from build123d import *

# Parameters (mm, degrees)
F0_R       = 8.5
F1_DEPTH   = 3
F2_SIZE2   = 3
F2_SIZE    = 1.45
F2_2_SIZE2 = 3
F2_2_SIZE  = 1.45
F2_3_SIZE2 = 3
F2_3_SIZE  = 1.45
F2_4_SIZE2 = 3
F2_4_SIZE  = 1.45
F2_5_SIZE2 = 3
F2_5_SIZE  = 1.45
F2_6_SIZE2 = 3
F2_6_SIZE  = 1.45
F2_7_SIZE2 = 3
F2_7_SIZE  = 1.45
F2_8_SIZE2 = 3
F2_8_SIZE  = 1.45
F3_SIZE2   = 1.45
F3_SIZE    = 3


with BuildPart() as f1:
    # F0 (on Top) → F1 (new body)
    with BuildSketch(Plane.XY):
        Polygon((9.5147186258, 10.9705627485), (-1.0294372515, 14.4852813742), (-10.9705627485, 9.5147186258), (-14.4852813742, -1.0294372515), (-9.5147186258, -10.9705627485), (1.0294372515, -14.4852813742), (10.9705627485, -9.5147186258), (14.4852813742, 1.0294372515), align=None)
        Circle(F0_R, mode=Mode.SUBTRACT)
        Polygon((-9.5147186258, -10.9705627485), (-14.4852813742, -1.0294372515), (-21.2132034356, -21.2132034356), (-10.6066017178, -10.6066017178), align=None)
        Polygon((1.0294372515, -14.4852813742), (-9.5147186258, -10.9705627485), (0, -30), (0, -15), align=None)
        Polygon((10.6066017178, -10.6066017178), (10.9705627485, -9.5147186258), (1.0294372515, -14.4852813742), (21.2132034356, -21.2132034356), align=None)
        Polygon((15, 0), (14.4852813742, 1.0294372515), (10.9705627485, -9.5147186258), (30, 0), align=None)
        Polygon((10.6066017178, 10.6066017178), (9.5147186258, 10.9705627485), (14.4852813742, 1.0294372515), (21.2132034356, 21.2132034356), align=None)
        Polygon((0, 30), (0, 15), (-1.0294372515, 14.4852813742), (9.5147186258, 10.9705627485), align=None)
        Polygon((-10.9705627485, 9.5147186258), (-1.0294372515, 14.4852813742), (-21.2132034356, 21.2132034356), (-10.6066017178, 10.6066017178), align=None)
        Polygon((-14.4852813742, -1.0294372515), (-10.9705627485, 9.5147186258), (-30, 0), (-15, 0), align=None)
    extrude(amount=F1_DEPTH)

    # F2
    f2_edges = [f1.edges().sort_by_distance(p)[0] for p in [
        (-15.909903, 15.909903, 3),
    ]]
    f2_side = f1.faces().sort_by_distance((-15.909903, 15.909903, 1.5))[0]
    chamfer(f2_edges, length=F2_SIZE, length2=F2_SIZE2, reference=f2_side)

    # F2#2
    f2_2_edges = [f1.edges().sort_by_distance(p)[0] for p in [
        (-22.5, 0, 3),
    ]]
    f2_2_side = f1.faces().sort_by_distance((-22.5, 0, 1.5))[0]
    chamfer(f2_2_edges, length=F2_2_SIZE, length2=F2_2_SIZE2, reference=f2_2_side)

    # F2#3
    f2_3_edges = [f1.edges().sort_by_distance(p)[0] for p in [
        (-15.909903, -15.909903, 3),
    ]]
    f2_3_side = f1.faces().sort_by_distance((-15.909903, -15.909903, 1.5))[0]
    chamfer(f2_3_edges, length=F2_3_SIZE, length2=F2_3_SIZE2, reference=f2_3_side)

    # F2#4
    f2_4_edges = [f1.edges().sort_by_distance(p)[0] for p in [
        (0, -22.5, 3),
    ]]
    f2_4_side = f1.faces().sort_by_distance((0, -22.5, 1.5))[0]
    chamfer(f2_4_edges, length=F2_4_SIZE, length2=F2_4_SIZE2, reference=f2_4_side)

    # F2#5
    f2_5_edges = [f1.edges().sort_by_distance(p)[0] for p in [
        (15.909903, -15.909903, 3),
    ]]
    f2_5_side = f1.faces().sort_by_distance((15.909903, -15.909903, 1.5))[0]
    chamfer(f2_5_edges, length=F2_5_SIZE, length2=F2_5_SIZE2, reference=f2_5_side)

    # F2#6
    f2_6_edges = [f1.edges().sort_by_distance(p)[0] for p in [
        (22.5, 0, 3),
    ]]
    f2_6_side = f1.faces().sort_by_distance((22.5, 0, 1.5))[0]
    chamfer(f2_6_edges, length=F2_6_SIZE, length2=F2_6_SIZE2, reference=f2_6_side)

    # F2#7
    f2_7_edges = [f1.edges().sort_by_distance(p)[0] for p in [
        (15.909903, 15.909903, 3),
    ]]
    f2_7_side = f1.faces().sort_by_distance((15.909903, 15.909903, 1.5))[0]
    chamfer(f2_7_edges, length=F2_7_SIZE, length2=F2_7_SIZE2, reference=f2_7_side)

    # F2#8
    f2_8_edges = [f1.edges().sort_by_distance(p)[0] for p in [
        (0, 22.5, 3),
    ]]
    f2_8_side = f1.faces().sort_by_distance((0, 22.5, 1.5))[0]
    chamfer(f2_8_edges, length=F2_8_SIZE, length2=F2_8_SIZE2, reference=f2_8_side)

    # F3
    f3_edges = [f1.edges().sort_by_distance(p)[0] for p in [
        (0, -22.5, 0),
        (15.909903, -15.909903, 0),
        (22.5, 0, 0),
        (15.909903, 15.909903, 0),
        (0, 22.5, 0),
        (-15.909903, 15.909903, 0),
        (-22.5, 0, 0),
        (-15.909903, -15.909903, 0),
    ]]
    f3_side = f1.faces().sort_by_distance((-16.509903, -15.309903, 0))[0]
    chamfer(f3_edges, length=F3_SIZE, length2=F3_SIZE2, reference=f3_side)


solid = f1.part
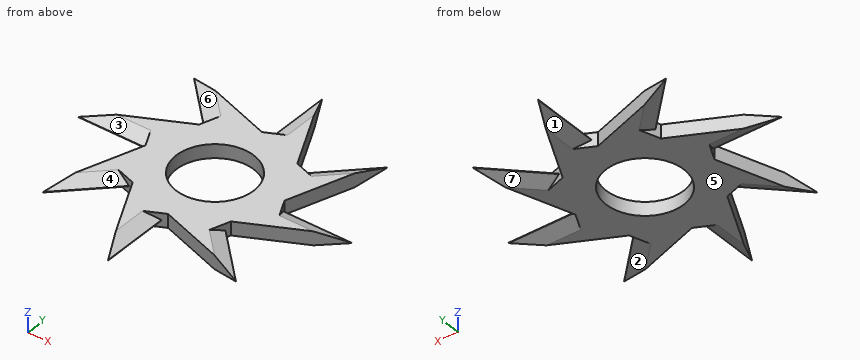
Here's how the part is built. I have some questions about the finished solid (model axes, mm). Face numbers are marked on the shaded views. A direction names the side the tool comes from. Give positions to 0.01 mm unless a question says otherwise; leave off trailing zeros. Order: outer loops, then holes, each group sorted by start corner. A loop starts at its lowest first (then second) coordinate and runs counter-clockwise, first axis right, second up. Notation, with made-up numbers: M 30,-24.75 L 61,-24.75 A25 ccw 61,9.25 Z; hole C -13.75,-13.75 d11. An arc over 180 degrees is marked long. Answer as a JSON object with one key per item and string values. Group by question number.
1) Suppose I cut it at C-C, the plane z = 2.25. Write out the boundary of the cut face in (x, y), plus the area to 3 significant figures.
2) Suppose I cut it at D-D, the plane x = -13. Write out the boundary of the cut face in (y, z), plus the area to 3 significant figures.
3) On a 3-axis mill with a long thin cutter (end or side, diameter ignored), from which of +Z, -Z, +X, -X, +Y, -Y can I reach the whole of each face in a straight line? I mean the marked faces 1, 2 and 3. Say none if no direction works.
4) Suppose I cut it at A-A, the plane x = -20. Write out the boundary of the cut face in (y, z), plus the area to 3 significant figures.
5) I'm going to push a flat-ended pin straight in: pin 1 Ø1.5 at (x, z) = (-4.5, 1) entering from -Y. Where does the tip first touch, or does it pass through?
6) Please list where these lines run through material, in increasing order: L1, parallel to Y at x = 0, z = 1.95; L2, parallel to X at y = -7.5, z = 0.7; L3, parallel to Z at x = -16.5, y = -14. Write a range as [from, to].
7) We'd pull the mould along Y, two halves only. Please class the marked faces 4, 5, 6 and 7: pulls with the +Y half, pulls with the -Y half, needs draft (parallel to the pull), parting line crosses it, or undercut.
8) Suppose I cut it at B-B, the plane y = -17.5. Write out the boundary of the cut face in (x, z), plus the area to 3 significant figures.
Results found:
{
 "1": {"outline": "M -27.1,1.45 L -15.72,1.45 L -14.49,-1.03 L -20.19,-18.14 L -12.14,-10.09 L -9.51,-10.97 L -1.45,-27.1 L -1.45,-15.72 L 1.03,-14.49 L 18.14,-20.19 L 10.09,-12.14 L 10.97,-9.51 L 27.1,-1.45 L 15.72,-1.45 L 14.49,1.03 L 20.19,18.14 L 12.14,10.09 L 9.51,10.97 L 1.45,27.1 L 1.45,15.72 L -1.03,14.49 L -18.14,20.19 L -10.09,12.14 L -10.97,9.51 Z; hole C 0,0 d17", "area": "824 mm²"},
 "2": {"outline": "M -13,1.45 L -9.81,0.36 L -9.81,0 L 8.5,0 L 8.5,3 L -9.81,3 L -9.81,2.64 L -13,1.55 Z; M 13,1.45 L 17.24,0 L 18.48,0 L 18.48,3 L 17.24,3 L 13,1.55 Z", "area": "69.0 mm²"},
 "3": {"face 1": "-Z, +Y", "face 2": "-Z, +X", "face 3": "+Z, -X"},
 "4": {"outline": "M -20,1.45 L -17.57,0.62 L -17.57,2.38 L -20,1.55 Z; M 0,1.45 L 3,0 L 5,0 L 5,3 L 3,3 L 0,1.55 Z; M 20,1.45 L 20.81,1.17 L 20.81,1.83 L 20,1.55 Z", "area": "13.2 mm²"},
 "5": {"pin 1": "y = -22.5"},
 "6": {"L1": "[-15, -8.5], [8.5, 15]", "L2": "[-16.64, -4], [4, 15]", "L3": "[0.6, 2.4]"},
 "7": {"face 4": "pulls with the -Y half", "face 5": "needs draft", "face 6": "undercut", "face 7": "pulls with the +Y half"},
 "8": {"outline": "M -19.98,0.6 L -17.5,1.45 L -17.5,1.55 L -19.98,2.4 Z; M -6.25,0 L -3,0 L 0,1.45 L 0,1.55 L -3,3 L -6.25,3 Z; M 10.07,0 L 13.26,0 L 17.5,1.45 L 17.5,1.55 L 13.26,3 L 10.07,3 Z", "area": "32.9 mm²"}
}
